Autodesk Inventor part; units mm, degrees
ref_plane "YZ Plane" through (0, 0, 0) normal (1, 0, 0) x (0, 1, 0)
ref_plane "XZ Plane" through (0, 0, 0) normal (0, 1, 0) x (-1, 0, 0)
ref_plane "XY Plane" through (0, 0, 0) normal (0, 0, 1) x (1, 0, 0)
sketch "Sketch1" plane through (0, 0, 0) normal (0, 0, 1) x (1, 0, 0)
  line L0 (-15, -17.5) -> (15, -17.5)
  line L1 (17.5, -15) -> (17.5, 15)
  line L2 (15, 17.5) -> (-15, 17.5)
  line L3 (-17.5, 15) -> (-17.5, -15)
  line L4 (-17.5, -17.5) -> (17.5, 17.5) construction
  line L5 (17.5, -17.5) -> (-17.5, 17.5) construction
  line L6 (-14.5, -14.5) -> (14.5, -14.5)
  line L7 (14.5, -14.5) -> (14.5, 14.5)
  line L8 (14.5, 14.5) -> (-14.5, 14.5)
  line L9 (-14.5, 14.5) -> (-14.5, -14.5)
  line L10 (-14.5, -14.5) -> (14.5, 14.5) construction
  line L11 (14.5, -14.5) -> (-14.5, 14.5) construction
  arc A0 (-15, 17.5) -> (-17.5, 15) centre (-15, 15) ccw
  arc A1 (17.5, 15) -> (15, 17.5) centre (15, 15) ccw
  arc A2 (15, -17.5) -> (17.5, -15) centre (15, -15) ccw
  arc A3 (-17.5, -15) -> (-15, -17.5) centre (-15, -15) ccw
  point P0 (0, 0)
  dimension "d0" = 35
  dimension "d1" = 35
  dimension "d2" = 29
  dimension "d3" = 29
  dimension "d4" = 2.5
extrude "Extrusion1" add sketch "Sketch1" along normal blind 150
sketch "Sketch2" plane through (-15, 17.5, 0) normal (0, 1, 0) x (1, 0, 0)
  line L0 (30, 0) -> (0, 0) construction
  line L1 (0, 0) -> (0, -150) construction
  line L2 (30, -150) -> (0, -150) construction
  line L3 (30, 0) -> (30, -150) construction
  line L4 (-2.5, 0) -> (-2.5, -150) construction
  line L5 (32.5, 0) -> (32.5, -150) construction
  line L6 (-7.5, 0) -> (32.5, 0)
  line L7 (-7.5, 0) -> (-7.5, -40)
  line L8 (-7.5, -40) -> (32.5, 0)
  line L9 (0, 0) -> (0, -150) construction
  line L10 (0, -75) -> (29.5, -75) construction
  line L11 (29.5, 0) -> (29.5, -150) construction
  line L12 (-7.5, -150) -> (32.5, -150)
  line L13 (-7.5, -150) -> (-7.5, -110)
  line L14 (-7.5, -110) -> (32.5, -150)
  point P0 (15, 0)
  dimension "d7" = 40
  dimension "d8" = 40
extrude "Extrusion2" cut sketch "Sketch2" against normal blind 100
sketch "Sketch5" plane through (15, 17.5, 147.5) normal (0, 1, 0) x (1, 0, 0)
  line L0 (-30, 30) -> (0, 0) construction
  line L1 (2.5, -2.5) -> (0, 0)
  line L2 (0, 0) -> (-42.4264, 42.4264) construction
  line L3 (-42.4264, 42.4264) -> (-63.6396, 21.2132)
  line L4 (-63.6396, 21.2132) -> (-21.2132, -21.2132)
  line L5 (-21.2132, -21.2132) -> (0, 0)
  line L6 (0, 145) -> (-30, 115) construction
  line L7 (0, 145) -> (2.5, 147.5)
  line L8 (0, 0) -> (0, 145)
  line L9 (-30, 115) -> (-30, 30) construction
  line L10 (-30, 72.5) -> (-0.5, 72.5) construction
  line L11 (-0.5, 144.5) -> (-0.5, 0.5) construction
  line L12 (0, 145) -> (-42.4264, 102.5736) construction
  line L13 (-42.4264, 102.5736) -> (-63.6396, 123.7868)
  line L14 (-63.6396, 123.7868) -> (-21.2132, 166.2132)
  line L15 (-21.2132, 166.2132) -> (0, 145)
  line L16 (-42.4264, 102.5736) -> (-42.4264, 42.4264)
  point P0 (-15, 147.5)
  dimension "d18" = 60
  dimension "d19" = 30
extrude "Extrusion5" add sketch "Sketch5" along normal blind 2
properties part number "TestPlate" material "Steel, Mild"
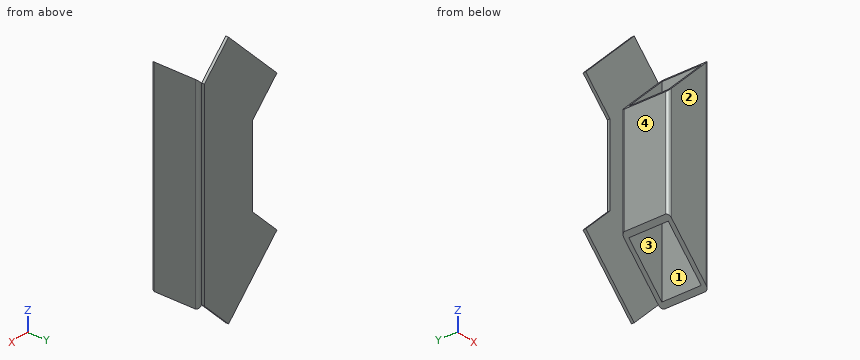
The listing builds one solid part. Answer for the finished solid, in the listing's coordinates (mm). Face numbers are marked on the shaded views. Give positions to 0.01 mm unless a question says otherwise; leave off trailing zeros. Write each loop counter-clockwise with the first axis right and the second up, starting at its lowest first coordinate (ties: lowest second). Pieces come first, ordered by that corner, then holes. Notation, with made-up numbers: M 63,24 L 113,24 A13 ccw 113,47 Z; hole C 64.5,-25 d5. An arc over 180 degrees is marked long. Write each question's results on one line, items separated by ' | '.
Q1. Flat-ended cylindrical pins translate along their axes: P1, Ø1.6, axis at y = 18.5, z = 89.5, coming from the -X side; P2, Ø8, axis at y = 12, z = 41.5, coming from the -X side; P3, Ø3, axis at x = 4, z = 143.5, coming from the -Y side. Find the tip coordinate at first contact, or state that the pin passes through.
Output values:
P1: x = -27.43 | P2: x = -17.5 | P3: y = 17.5
Q2. Consider L1, parallel to X at y = 13, z = 107.5; L2, parallel to Y at x = 13, z = 107.5; L3, parallel to Y at x = -6, z = 7. Determine where each line is inside the solid, lowest interval first. Write a range as from..to.
Output values:
L1: -17.5..-14.5, 14.5..17.5 | L2: -17.5..-14.5, 14.5..19.5 | L3: 17.5..19.5
Q3. For a pull along Y with two mould halves and no side action, classify the marked faces 1, 2, 3 and 4 as released by +Y, released by -Y, zero draft, split by the parting line, or undercut.
Output values:
face 1: undercut | face 2: released by -Y | face 3: undercut | face 4: zero draft
Q4. Section D-D, the plane x = 10 is taken. Write down the section's boundary in (y, z).
Output values:
outline: M -17.5,7.5 L -14.5,7.5 L -14.5,142.5 L -17.5,142.5 Z; M 14.5,7.5 L 17.5,7.5 L 17.5,-2.5 L 19.5,-2.5 L 19.5,152.5 L 17.5,152.5 L 17.5,142.5 L 14.5,142.5 Z
Q5. Section C-C, the plane z = 103 is taken. Write down the section's boundary in (x, y), then the cut area to 3 significant figures.
Output values:
outline: M -27.43,17.5 L -15,17.5 A2.5 ccw -17.5,15 L -17.5,-15 A2.5 ccw -15,-17.5 L 15,-17.5 A2.5 ccw 17.5,-15 L 17.5,15 A2.5 ccw 15,17.5 L 15,19.5 L -27.43,19.5 Z; hole M -14.5,-14.5 L 14.5,-14.5 L 14.5,14.5 L -14.5,14.5 Z | area: 463 mm2
Q6. Section A-A, the plane x = 2 is taken. Write down the section's boundary in (y, z), then the cut area to 3 significant figures.
Output values:
outline: M -17.5,15.5 L -14.5,15.5 L -14.5,134.5 L -17.5,134.5 Z; M 14.5,15.5 L 17.5,15.5 L 17.5,-10.5 L 19.5,-10.5 L 19.5,160.5 L 17.5,160.5 L 17.5,134.5 L 14.5,134.5 Z | area: 1,060 mm2
Q7. Section B-B, the plane y = 12.5 is taken. Write down the section's boundary in (x, z), then the cut area to 3 significant figures.
Output values:
outline: M -17.5,35 L -14.5,32 L -14.5,118 L -17.5,115 Z; M 14.5,3 L 17.5,0 L 17.5,150 L 14.5,147 Z | area: 690 mm2
